CAD build for the part. Positions are in the model's coordinates, mm. Round coordinates to 2 decimals unless told otherwise and drop trailing zeros. Order: outer loops, then holes, each group sorted by start corner. A loop starts at its lowest first (then second) coordinate and runs counter-clockwise, first axis right, second up. Notation, with made-up numbers: M -30,66 L 0,66 A31 cw 0,99 Z; hole C -15.75,68 d8. An arc over 180 degrees is marked long. Put each result on its own line as item: value.
Autodesk Inventor part; units mm, degrees
ref_plane "YZ Plane" through (0, 0, 0) normal (1, 0, 0) x (0, 1, 0)
ref_plane "XZ Plane" through (0, 0, 0) normal (0, 1, 0) x (-1, 0, 0)
ref_plane "XY Plane" through (0, 0, 0) normal (0, 0, 1) x (1, 0, 0)
sketch "Sketch1" plane through (0, 0, 0) normal (0, 1, 0) x (-1, 0, 0)
  line L0 (10, -7.5) -> (-10, -7.5)
  line L1 (-10, -7.5) -> (-10, 7.5)
  line L2 (-10, 7.5) -> (10, 7.5)
  line L3 (10, 7.5) -> (10, -7.5)
  line L4 (14, 0) -> (-14, 0)
  line L5 (0, -10.5) -> (0, 10.5)
  point P0 (0, 0)
  dimension "d0" = 15
  dimension "d1" = 20
extrude "Extrusion1" add sketch "Sketch1" along normal blind 10
sketch "Sketch2" plane through (10, 0, 7.5) normal (1, 0, 0) x (0, 0, -1)
  line L0 (0, 0) -> (15, 0)
  line L1 (15, 0) -> (15, 10)
  line L2 (0, 10) -> (15, 10)
  line L3 (0, 0) -> (0, 10)
  circle A0 centre (7.5, 5) radius 2.5
  line L4 (15, 10) -> (0, 0) construction
  line L5 (0, 10) -> (15, 0) construction
  point P0 (7.5, 0)
  dimension "d4" = 5
extrude "Extrusion2" cut sketch "Sketch2" against normal through all contours A0
properties part number "stop_block"
Item 1: Band-saw the part on B-B on y = 5. Give the cut face in (x, z), and give its area (3 significant figures).
Answers below:
outline: M -10,-7.5 L 10,-7.5 L 10,-2.5 L -10,-2.5 Z; M -10,2.5 L 10,2.5 L 10,7.5 L -10,7.5 Z
area: 200 mm²
Item 2: Pin check, flat tip, straight feed: P1, Ø6, axis at y = 5, z = 0, coming from the -X side. Stop position of the tip, or through.
Answers below:
P1: x = -10
Item 3: Probe line 1 along Y through (x, z) = (3, 0); line 2 along Y through (x, z) = (-6.25, 1.5); line 3 along Z through (x, y) = (-1, 3.5). List the from-to ranges inside material, lowest first. Write a range as [from, to].
Answers below:
line 1: [0, 2.5], [7.5, 10]
line 2: [0, 3], [7, 10]
line 3: [-7.5, -2], [2, 7.5]
Item 4: Mould opens along Z. For faces 1 (the flat face through (0, 5, 7.5)), 2 (the cylindrical face through (0.14, 7.48, 0.33)), 3 (the flat face through (-10, 3, 2)) say: pulls with the +Z half, pulls with the -Z half, needs draft (parallel to the pull), parting line crosses it, or undercut.
Answers below:
face 1: pulls with the +Z half
face 2: undercut
face 3: needs draft
Item 5: Band-saw the part on C-C on x = 0. Give the cut face in (y, z).
Answers below:
outline: M 0,-7.5 L 10,-7.5 L 10,7.5 L 0,7.5 Z; hole C 5,0 d5
Item 6: Band-saw the part on A-A on z = 0. Give the cut face in (x, y), and give its area (3 significant figures).
Answers below:
outline: M -10,0 L 10,0 L 10,2.5 L -10,2.5 Z; M -10,7.5 L 10,7.5 L 10,10 L -10,10 Z
area: 100 mm²
